from build123d import *

# Parameters (mm, degrees)
F0_R     = 5
F1_DEPTH = 11
F2_W     = 920
F2_H     = 754.619706
F3_DEPTH = 7
F4_R     = 5
F5_DEPTH = 11


with BuildPart() as f1:
    # F0 (on Top) → F1 (new body)
    with BuildSketch(Plane.XY):
        with BuildLine():
            Line((461.123695, 406.42578), (-458.876305, 406.42578))
            Line((-458.876305, 406.42578), (-458.876305, -348.193926))
            Line((-458.876305, -348.193926), (-425.832388, -348.193926))
            Line((-425.832388, -348.193926), (-425.875983, -333.799931))
            ThreePointArc((-425.875983, -333.799931), (-425.876224, -333.746929), (-425.876305, -333.693926))
            ThreePointArc((-425.876305, -333.693926), (-408.376305, -316.193926), (-390.876305, -333.693926))
            Line((-390.876305, -333.693926), (-390.876305, -348.193926))
            Line((-390.876305, -348.193926), (391.123695, -348.193926))
            Line((391.123695, -348.193926), (391.123695, -333.693926))
            ThreePointArc((391.123695, -333.693926), (408.623695, -316.193926), (426.123695, -333.693926))
            Line((426.123695, -333.693926), (426.123695, -348.193926))
            Line((426.123695, -348.193926), (461.123695, -348.193926))
            Line((461.123695, -348.193926), (461.123695, 406.42578))
        make_face()
        with Locations((-408.429307, -303.193926)):
            Circle(F0_R, mode=Mode.SUBTRACT)
        with Locations((408.623695, -303.193926)):
            Circle(F0_R, mode=Mode.SUBTRACT)
    extrude(amount=F1_DEPTH)

    # F2 (on face) → F3 (join)
    with BuildSketch(Plane.XY.offset(11)):
        with Locations((1.123695, 29.115927)):
            Rectangle(F2_W, F2_H)
    extrude(amount=F3_DEPTH)

    # F4 (on face) → F5 (cut)
    with BuildSketch(Plane(origin=(0, 0, 0), x_dir=(1, 0, 0), z_dir=(0, 0, -1))):
        with BuildLine():
            Line((-75.876305, 348.193926), (-75.876305, 333.713589))
            ThreePointArc((-75.876305, 333.713589), (-58.106118, 316.196012), (-40.885277, 334.25391))
            Line((-40.885277, 334.25391), (-40.885277, 348.193926))
            Line((-40.885277, 348.193926), (-56.401658, 373.656452))
            Line((-56.401658, 373.656452), (-75.876305, 348.193926))
        make_face()
        with Locations((-58.376316, 303.193926)):
            Circle(F4_R)
    extrude(amount=-F5_DEPTH, mode=Mode.SUBTRACT)


solid = f1.part
Input: part model. Units: mm. Frame: model coordinates. A direction names the side the tool comes from. Give positions to 0.01 mm unless a question says otherwise; leave off trailing zeros. Use CSV: the item, a comma, the result in double quotes. Start each with the question number.
Item 1: Line query: line 1 (Y direction, x = -392.5, z = 4); line 2 (Y direction, x = 394.5, z = 7.75). Output: solid intervals per line, ascending.
Item 2: Mould query, pull axis X, two halves, no side actions, for faces 3 (the flat face through (-59, -332, 11)), 4 (the flat face through (-5, 34, 18)), 5 (the flat face through (-458.876, 24, 9)). Classes: pulls with the +X half, pulls with the -X half, needs draft (parallel to the pull), parting line crosses it, or undercut.
Item 3: Reachability of faces 1 (the flat face through (-5, 34, 0)), 2 (the flat face through (-409, -332, 11)) from +Z, -Z, +X, -X, +Y, -Y: full face, straight path, thin tool, end or side. Return the list, or none.
Item 4: Contact query for a flat-ended pin moving along its axis: P1, Ø6, axis at x = 408.62, y = -303.19, coming from the -Z side. Output: stop coordinate, or through.
Ans:
1,line 1,"y = -326.33 to 406.43"
1,line 2,"y = -323.36 to 406.43"
2,face 3,"undercut"
2,face 4,"needs draft"
2,face 5,"pulls with the -X half"
3,face 1,"-Z, +X, -X, +Y, -Y"
3,face 2,"-Z, -Y"
4,P1,"stops at z = 11"
